from build123d import *

# Parameters (mm, degrees)
F0_R      = 15
F1_DEPTH  = 7
F2_R      = 14
F3_DEPTH  = 5
F4_R      = 6.167621
F5_DEPTH  = 5
F6_R      = 5
F7_DEPTH  = 3.5
F8_R      = 3.5
F9_DEPTH  = 3.5
F11_DEPTH = 2


with BuildPart() as f1:
    # F0 (on Top) → F1 (new body)
    with BuildSketch(Plane.XY):
        Circle(F0_R)
    extrude(amount=F1_DEPTH)

    # F2 (on face) → F3 (cut)
    with BuildSketch(Plane.XY.offset(7)):
        Circle(F2_R)
    extrude(amount=-F3_DEPTH, mode=Mode.SUBTRACT)

    # F4 (on face) → F5 (join)
    with BuildSketch(Plane.XY.offset(2)):
        Circle(F4_R)
    extrude(amount=F5_DEPTH)

    # F6 (on face) → F7 (cut)
    with BuildSketch(Plane.XY.offset(7)):
        Circle(F6_R)
    extrude(amount=-F7_DEPTH, mode=Mode.SUBTRACT)

    # F8 (on face) → F9 (cut, through all)
    with BuildSketch(Plane.XY.offset(3.5)):
        Circle(F8_R)
    extrude(amount=-F9_DEPTH, mode=Mode.SUBTRACT)

    # F10 (on face) → F11 (cut, through all)
    with BuildSketch(Plane.XY.offset(2)):
        Polygon((0.968024, 13.966493), (4.361166, 4.361166), (13.966493, 0.968024), (9.899495, 9.899495), align=None)
        Polygon((-13.966493, 0.968024), (-4.361166, 4.361166), (-0.968024, 13.966493), (-9.899495, 9.899495), align=None)
        Polygon((-0.968024, -13.966493), (-4.361166, -4.361166), (-13.966493, -0.968024), (-9.899495, -9.899495), align=None)
        Polygon((13.966493, -0.968024), (4.361166, -4.361166), (0.968024, -13.966493), (9.899495, -9.899495), align=None)
    extrude(amount=-F11_DEPTH, mode=Mode.SUBTRACT)


solid = f1.part
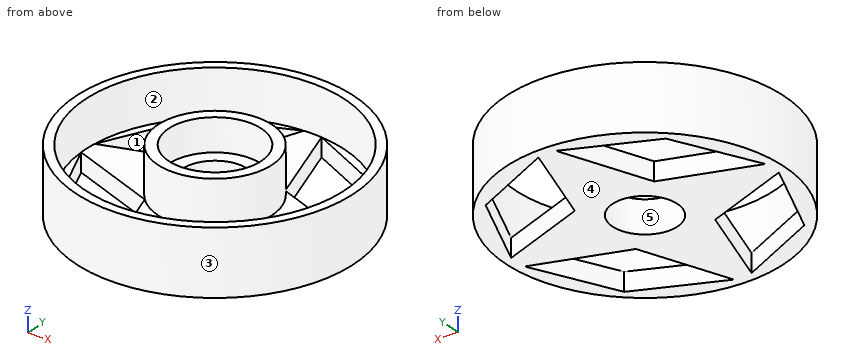
Design review of the part built by this model. Coordinates are the model's own, in mm. Face numbers are marked on the shaded views. A direction names the side the tool comes from. Round coordinates to 2 decimals unless told otherwise and drop trailing zeros. Write each loop counter-clockwise with the first axis right and the second up, starting at its lowest first coordinate (ties: lowest second). Pieces come first, ordered by that corner, then holes.
Item 1: Draft analysis for pull direction Y (two halves, no side actions). For the marked faces 3, 4 and 5, state which applies: released by +Y, released by -Y, zero draft, split by the parting line, or undercut.
Item 2: Consider section D-D on x = 7.75. Give the boundary of the cut face in (y, z), and give its area (4 significant figures).
Item 3: Consider section C-C on y = 8. Give the boundary of the cut face in (x, z), and give its area (3 significant figures).
Item 4: For the marked faces 1 and 2, list the 3-axis set-ups (+Z, -Z, +X, -X, +Y, -Y) from which the entire face can be reached by the end or side of a thin tool; tool diameter is ignored.
Item 5: Consider section A-A on x = 0. Give the boundary of the cut face in (y, z), and give its area (3 significant figures).
Item 6: Wall thickness on L1, parallel to Y at x = 0, z = 6.2; L2, parallel to Y at x = 4, z = 5.5; L3, parallel to Y at x = 6.5, z = 1.25: over which ranges is each line inside the solid? List them lowest first.
Item 7: For pin 1 Ø1.5 at (x, z) = (11.5, 3) entering from -Y; pin 2 Ø1 at (y, z) = (3.5, 3.5) entering from +X; pin 3 Ø6 at (x, y) = (0, 0) entering from -Z; pin 4 Ø1.2 at (x, y) = (-11.5, 6) entering from +Z, all flat-tipped, find the tip position at first contact; note any pin that passes through.
Check values:
1. face 3: split by the parting line
1. face 4: zero draft
1. face 5: undercut
2. outline: (-12.84, 0) - (-10.88, 0) - (-10.88, 2) - (-11.66, 2) - (-11.66, 7) - (-12.84, 7) - close; (-3.16, 0) - (3.16, 0) - (3.16, 2) - (-3.16, 2) - close; (10.88, 0) - (12.84, 0) - (12.84, 7) - (11.66, 7) - (11.66, 2) - (10.88, 2) - close
2. area: 32.35 mm2
3. outline: (-12.69, 0) - (-10.76, 0) - (-10.76, 2) - (-11.49, 2) - (-11.49, 7) - (-12.69, 7) - close; (-3.08, 0) - (3.08, 0) - (3.08, 2) - (-3.08, 2) - close; (10.76, 0) - (12.69, 0) - (12.69, 7) - (11.49, 7) - (11.49, 2) - (10.76, 2) - close
3. area: 32.0 mm2
4. face 1: +Z, -Z
4. face 2: +Z
5. outline: (-15, 0) - (-3.5, 0) - (-3.5, 3.5) - (-5, 3.5) - (-5, 7) - (-6.17, 7) - (-6.17, 2) - (-14, 2) - (-14, 7) - (-15, 7) - close; (3.5, 0) - (15, 0) - (15, 7) - (14, 7) - (14, 2) - (6.17, 2) - (6.17, 7) - (5, 7) - (5, 3.5) - (3.5, 3.5) - close
5. area: 72.2 mm2
6. L1: y = -15 to -14, -6.17 to -5, 5 to 6.17, 14 to 15
6. L2: y = -14.46 to -13.42, -4.69 to -3, 3 to 4.69, 13.42 to 14.46
6. L3: y = -13.52 to -11.45, -3.61 to 3.61, 11.45 to 13.52
7. pin 1: stops at y = -10.46
7. pin 2: stops at x = 14.7
7. pin 3: passes through
7. pin 4: stops at z = 2
